```python
from build123d import *

# Parameters (mm, degrees)
SKETCH070_W     = 177
SKETCH070_H     = 100
PAD042_DEPTH    = 48
POCKET026_DEPTH = 46
SKETCH072_W     = 11
SKETCH072_H     = 46.5
SKETCH072_W_2   = 11.5
POCKET027_DEPTH = 5
SKETCH075_W     = 8.1
SKETCH075_H     = 9.5
PAD045_DEPTH    = 4.3
SKETCH077_R     = 1.15
POCKET029_DEPTH = 3
SKETCH086_R     = 3.3
SKETCH086_R_2   = 1.15
PAD052_DEPTH    = 4
SKETCH088_W     = 4
SKETCH088_H     = 6
SKETCH088_W_2   = 30.4
SKETCH088_H_2   = 2.5
POCKET032_DEPTH = 5
SKETCH089_W     = 13.5
SKETCH089_H     = 10
SKETCH089_W_2   = 16
SKETCH089_H_2   = 8
SKETCH089_W_3   = 7
SKETCH089_H_3   = 6
SKETCH089_W_4   = 9
POCKET033_DEPTH = 5
PAD054_DEPTH    = 15
POCKET034_DEPTH = 5
SKETCH092_R     = 1.15
POCKET035_DEPTH = 5
SKETCH093_W     = 95.5
SKETCH093_H     = 46.5
PAD055_DEPTH    = 0.5
SKETCH094_W     = 11
SKETCH094_H     = 31
SKETCH094_W_2   = 4.3
PAD056_DEPTH    = 10


with BuildPart() as part:
    # Sketch070 → Pad042 (new body)
    with BuildSketch(Plane.XZ):
        Rectangle(SKETCH070_W, SKETCH070_H)
    extrude(amount=-PAD042_DEPTH)

    # Sketch071 (on Face6 of Pad042) → Pocket026 (cut)
    with BuildSketch(Plane(origin=(0, 48, 0), x_dir=(1, 0, 0), z_dir=(0, 1, 0))):
        Polygon((-86.5, 48), (-86.5, -48), (-75.5, -48), (-75.5, -50), (-64.5, -50), (-64.5, -48), (35.7, -48), (35.7, -50), (42.2, -50), (42.2, -48), (64.2, -48), (64.2, -50), (75.2, -50), (75.2, -48), (86.5, -48), (86.5, 48), align=None)
    extrude(amount=-POCKET026_DEPTH, mode=Mode.SUBTRACT)

    # Sketch072 (on Face6 of Pocket026) → Pocket027 (cut)
    with BuildSketch(Plane(origin=(0, 2, 0), x_dir=(1, 0, 0), z_dir=(0, 1, 0))):
        Polygon((64.5, -50), (75.2, -50), (75.2, -3.5), (64.5, -3.5), (64.5, -27), (59.5, -27), (59.5, -33), (64.5, -33), align=None)
        with Locations((-70, -26.75)):
            Rectangle(SKETCH072_W, SKETCH072_H)
        with Locations((36.75, -26.75)):
            Rectangle(SKETCH072_W_2, SKETCH072_H)
    extrude(amount=-POCKET027_DEPTH, mode=Mode.SUBTRACT)

    # Sketch075 (on Face20 of Pocket027) → Pad045 (join)
    with BuildSketch(Plane(origin=(0, 2, 0), x_dir=(1, 0, 0), z_dir=(0, 1, 0))):
        with Locations((62.65, 1.25)):
            Rectangle(SKETCH075_W, SKETCH075_H)
        with Locations((-62.55, 1.25)):
            Rectangle(SKETCH075_W, SKETCH075_H)
    extrude(amount=PAD045_DEPTH)

    # Sketch077 (on Face42 of Pad045) → Pocket029 (cut)
    with BuildSketch(Plane(origin=(0, 6.3, 0), x_dir=(1, 0, 0), z_dir=(0, 1, 0))):
        with Locations((64, 1)):
            Circle(SKETCH077_R)
        with Locations((-64, 1)):
            Circle(SKETCH077_R)
    extrude(amount=-POCKET029_DEPTH, mode=Mode.SUBTRACT)

    # Sketch086 (on Face23 of Pocket029) → Pad052 (join)
    with BuildSketch(Plane(origin=(0, 2, 0), x_dir=(1, 0, 0), z_dir=(0, 1, 0))):
        with Locations((7, 2.3)):
            Circle(SKETCH086_R)
        with Locations((7, 2.3)):
            Circle(SKETCH086_R_2, mode=Mode.SUBTRACT)
        with Locations((25, 2.3)):
            Circle(SKETCH086_R)
        with Locations((25, 2.3)):
            Circle(SKETCH086_R_2, mode=Mode.SUBTRACT)
        with Locations((7, -19.2)):
            Circle(SKETCH086_R)
        with Locations((7, -19.2)):
            Circle(SKETCH086_R_2, mode=Mode.SUBTRACT)
        with Locations((25, -19.2)):
            Circle(SKETCH086_R)
        with Locations((25, -19.2)):
            Circle(SKETCH086_R_2, mode=Mode.SUBTRACT)
        with Locations((-77.5, 39)):
            Circle(SKETCH086_R)
        with Locations((-77.5, 39)):
            Circle(SKETCH086_R_2, mode=Mode.SUBTRACT)
        with Locations((77.5, 39)):
            Circle(SKETCH086_R)
        with Locations((77.5, 39)):
            Circle(SKETCH086_R_2, mode=Mode.SUBTRACT)
        with Locations((77.5, 14)):
            Circle(SKETCH086_R)
        with Locations((77.5, 14)):
            Circle(SKETCH086_R_2, mode=Mode.SUBTRACT)
        with Locations((-77.5, 14)):
            Circle(SKETCH086_R)
        with Locations((-77.5, 14)):
            Circle(SKETCH086_R_2, mode=Mode.SUBTRACT)
        with Locations((-57.5, -33)):
            Circle(SKETCH086_R)
        with Locations((-57.5, -33)):
            Circle(SKETCH086_R_2, mode=Mode.SUBTRACT)
        with Locations((-7, -33)):
            Circle(SKETCH086_R)
        with Locations((-7, -33)):
            Circle(SKETCH086_R_2, mode=Mode.SUBTRACT)
    extrude(amount=PAD052_DEPTH)

    # Sketch088 (on Face39 of Pad052) → Pocket032 (cut)
    with BuildSketch(Plane(origin=(0, 0, 48), x_dir=(1, 0, 0), z_dir=(0, 0, -1))):
        with Locations((62.2, -5)):
            Rectangle(SKETCH088_W, SKETCH088_H)
        with Locations((-41.48, -24.98)):
            Rectangle(SKETCH088_W_2, SKETCH088_H_2)
    extrude(amount=-POCKET032_DEPTH, mode=Mode.SUBTRACT)

    # Sketch089 (on Face22 of Pocket032) → Pocket033 (cut)
    with BuildSketch(Plane(origin=(0, 0, -50), x_dir=(1, 0, 0), z_dir=(0, 0, -1))):
        with Locations((52.75, -13)):
            Rectangle(SKETCH089_W, SKETCH089_H)
        with Locations((-21.2, -12)):
            Rectangle(SKETCH089_W_2, SKETCH089_H_2)
        with Locations((25.2, -11)):
            Rectangle(SKETCH089_W_3, SKETCH089_H_3)
        with Locations((11.5, -11)):
            Rectangle(SKETCH089_W_4, SKETCH089_H_3)
    extrude(amount=-POCKET033_DEPTH, mode=Mode.SUBTRACT)

    # Sketch090 (on Face4 of Pocket033) → Pad054 (join)
    with BuildSketch(Plane(origin=(0, 48, 0), x_dir=(1, 0, 0), z_dir=(0, 1, 0))):
        with BuildLine():
            Line((-86.5, -48), (-79.5, -48))
            Line((-79.5, -48), (-79.5, -39))
            ThreePointArc((-79.5, -39), (-81.550253, -34.050253), (-86.5, -32))
            Line((-86.5, -32), (-86.5, -39))
            Line((-86.5, -39), (-86.5, -48))
        make_face()
        with BuildLine():
            Line((86.5, -48), (86.5, -39))
            Line((86.5, -32), (86.5, -39))
            ThreePointArc((86.5, -32), (81.550253, -34.050253), (79.5, -39))
            Line((79.5, -39), (79.5, -48))
            Line((79.5, -48), (86.5, -48))
        make_face()
        with BuildLine():
            Line((-86.5, 48), (-86.5, 39))
            Line((-86.5, 39), (-86.5, 32))
            ThreePointArc((-86.5, 32), (-81.550253, 34.050253), (-79.5, 39))
            Line((-79.5, 39), (-79.5, 48))
            Line((-79.5, 48), (-86.5, 48))
        make_face()
        with BuildLine():
            Line((86.5, 48), (79.5, 48))
            Line((79.5, 48), (79.5, 39))
            ThreePointArc((79.5, 39), (81.550253, 34.050253), (86.5, 32))
            Line((86.5, 39), (86.5, 32))
            Line((86.5, 39), (86.5, 48))
        make_face()
    extrude(amount=-PAD054_DEPTH)

    # Sketch091 (on Face38 of Pad054) → Pocket034 (cut)
    with BuildSketch(Plane(origin=(0, 48, 0), x_dir=(1, 0, 0), z_dir=(0, 1, 0))):
        with BuildLine():
            Line((-86.5, 32), (-86.5, 48))
            Line((-86.5, 48), (-79.5, 48))
            Line((-79.5, 48), (-79.5, 39))
            ThreePointArc((-86.5, 32), (-81.550253, 34.050253), (-79.5, 39))
        make_face()
        with BuildLine():
            Line((79.5, 48), (86.5, 48))
            Line((86.5, 48), (86.5, 32))
            ThreePointArc((79.5, 39), (81.550253, 34.050253), (86.5, 32))
            Line((79.5, 48), (79.5, 39))
        make_face()
        with BuildLine():
            ThreePointArc((-79.5, -39), (-81.550253, -34.050253), (-86.5, -32))
            Line((-86.5, -48), (-86.5, -32))
            Line((-79.5, -48), (-86.5, -48))
            Line((-79.5, -39), (-79.5, -48))
        make_face()
        with BuildLine():
            Line((79.5, -48), (86.5, -48))
            Line((86.5, -48), (86.5, -32))
            ThreePointArc((86.5, -32), (81.550253, -34.050253), (79.5, -39))
            Line((79.5, -48), (79.5, -39))
        make_face()
    extrude(amount=-POCKET034_DEPTH, mode=Mode.SUBTRACT)

    # Sketch092 (on Face110 of Pocket034) → Pocket035 (cut)
    with BuildSketch(Plane(origin=(0, 43, 0), x_dir=(1, 0, 0), z_dir=(0, 1, 0))):
        with Locations((83, -43.5)):
            Circle(SKETCH092_R)
        with Locations((-83, -43.5)):
            Circle(SKETCH092_R)
        with Locations((-83, 43.5)):
            Circle(SKETCH092_R)
        with Locations((83, 43.5)):
            Circle(SKETCH092_R)
    extrude(amount=-POCKET035_DEPTH, mode=Mode.SUBTRACT)

    # Sketch093 (on Face2 of Pocket035) → Pad055 (join)
    with BuildSketch(Plane.XZ):
        with Locations((-16.75, 26.75)):
            Rectangle(SKETCH093_W, SKETCH093_H)
        Polygon((64.5, 50), (75.2, 50), (75.2, 3.5), (64.5, 3.5), (64.5, 22), (69.5, 22), (69.5, 33), (64.5, 33), align=None)
    extrude(amount=-PAD055_DEPTH)

    # Sketch094 (on Face70 of Pad055) → Pad056 (join)
    with BuildSketch(Plane(origin=(0, 0, 48), x_dir=(1, 0, 0), z_dir=(0, 0, -1))):
        Polygon((-64.5, -44), (-57.5, -44), (-57.5, -42), (-62.5, -42), (-62.5, -17), (-64.5, -17), align=None)
        Polygon((64.2, -44), (57.2, -44), (57.2, -42), (62.2, -42), (62.2, -33), (64.2, -33), align=None)
        with Locations((-81, -17.5)):
            Rectangle(SKETCH094_W, SKETCH094_H)
        with Locations((77.35, -17.5)):
            Rectangle(SKETCH094_W_2, SKETCH094_H)
    extrude(amount=PAD056_DEPTH)


with BuildPart() as part_1:
    # Body018 placement: moved
    add(part.part.moved(Location((0, -52, -56))))


solid = part_1.part
```
Model file for the job. Use its own axes, mm. A direction names the side the tool comes from. Coordinates: 2 decimals unless noted, no trailing zeros. Loops run counter-clockwise (first coordinate to the right, second up) from the corner with the lowest first, then second, coordinate; pieces in that order, holes last. Notation, with made-up numbers: (-9, -16) -> (12, -16) arc R14 cw to (12, 10) -> close; hole circle Ø7 at (43.5, 84). An arc over 180 degrees is marked (long way). Answer as a JSON object with one key per item and string values.
Q1. Probe probe 1 along X at (y, z) = (-47, -23); probe 2 along X at (y, z) = (-11.1, -99.5); probe 3 along X at (y, z) = (-49.05, -36.8). List the from-to ranges inside material, lowest first.
Report:
{"probe 1": "x = -88.5 to -86.5, -60.8 to -58.65, -56.35 to -54.2, -10.3 to -8.15, -5.85 to -3.7, 86.5 to 88.5", "probe 2": "x = -88.5 to -84.15, -81.85 to -79.5, 79.5 to 81.85, 84.15 to 88.5", "probe 3": "x = -88.5 to -86.5, 3.7 to 5.85, 8.15 to 10.3, 21.7 to 23.85, 26.15 to 28.3, 86.5 to 88.5"}
Q2. Cut at A-A (y = -31). List the corners of the cut face in (x, z).
Report:
{"outline": "(-88.5, -106) -> (88.5, -106) -> (88.5, -6) -> (75.2, -6) -> (75.2, -18) -> (79.5, -18) -> (79.5, -8) -> (86.5, -8) -> (86.5, -104) -> (-86.5, -104) -> (-86.5, -18) -> (-75.5, -18) -> (-75.5, -6) -> (-88.5, -6) -> close; (-64.5, -18) -> (-62.5, -18) -> (-62.5, -8) -> (35.7, -8) -> (35.7, -6) -> (-64.5, -6) -> close; (42.2, -8) -> (64.2, -8) -> (64.2, -6) -> (42.2, -6) -> close"}
Q3. Flat gauge pins, fed straight in: P1, Ø0.7, axis at x = -7, z = -23, coming from the +Y side; P2, Ø9, axis at x = -63, z = -57, coming from the +Y side; P3, Ø1.5, axis at x = -66, y = -34.5, coming from the +Z side. Where does each tip first touch, or does it go through?
Report:
{"P1": "stops at y = -50", "P2": "stops at y = -45.7", "P3": "stops at z = -104"}
Q4. Pull direction Y, two halves, no side cores. Call faces 4 (the cylindrical face through (75.07, -48.03, -97.23)), 5 (the flat face through (-1, -52, -55)), 6 (the flat face through (-65, -49, -52.5)): released by +Y, released by -Y, zero draft, split by the parting line, or undercut.
Report:
{"face 4": "undercut", "face 5": "released by -Y", "face 6": "zero draft"}
Q5. 3-axis set-ups, long thin cutter, end or side, ignore diameter. For faces 1 (the flat face through (-78, -19, -13)), 2 (the flat face through (62.2, -14, -13)), 3 (the flat face through (-66.6, -48, -57)): which of +Z, -Z, +X, -X, +Y, -Y reach the whole face in a straight line?
Report:
{"face 1": "+Y", "face 2": "none", "face 3": "+Z, +Y"}
